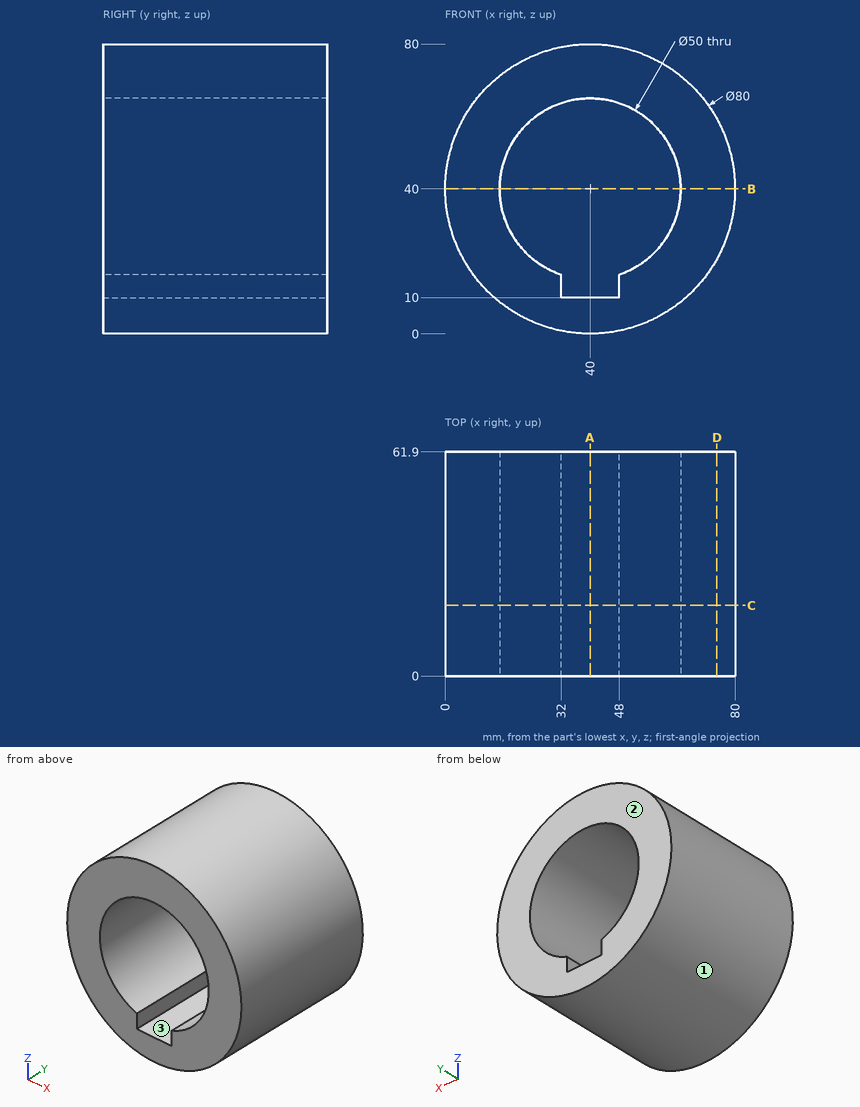
Print and shaded views of the part. All mm, measured from the part's lowest x, y and z. Coordinates: 2 decimals unless noted, no trailing zeros. Write each loop counter-clockwise with the first axis right and the second up, starting at its lowest first coordinate (ties: lowest second). Pieces come first, ordered by that corner, then holes.
(1) Cut at A-A, the plane x = 40. List the corners of the cut face in (y, z).
(2) Cut at D-D, the plane x = 75. List the corners of the cut face in (y, z).
(3) Drill centre lines: probe 1 along X at (y, z) = (45.5, 40); probe 2 along X at (y, z) = (14, 51); probe 3 along Z at (x, y) = (27.5, 32). Where is each one in solid material? Low to high.
(4) Two-plate mould, pull along Z, no slides. Class the marked faces 1, 2 and 3: +Z half, -Z half, draft (parallel to the pull), parting line (faces both ways), or undercut.
(5) Flat gauge pins, fed straight in: pin 1 (1.5 mm diameter, centred on y = 27, z = 25.5, fed in from +X); pin 2 (8 mm diameter, centred on x = 29, y = 46, fed in from -Z); pin 3 (10 mm diameter, centred on y = 39.5, z = 63, fed in from +X). Where does each tip first touch, or does it go through?
(6) Cut at C-C, the plane y = 19.5. List the corners of the cut face in (x, z), and give its area (3 significant figures).
(7) Cut at B-B, the plane z = 40. List the corners of the cut face in (x, y).
Geometry says:
1. outline: (0, 0) - (61.9, 0) - (61.9, 10) - (0, 10) - close; (0, 65) - (61.9, 65) - (61.9, 80) - (0, 80) - close
2. outline: (0, 20.64) - (61.9, 20.64) - (61.9, 59.36) - (0, 59.36) - close
3. probe 1: x = 0 to 15, 65 to 80
3. probe 2: x = 1.54 to 17.55, 62.45 to 78.46
3. probe 3: z = 2 to 18.35, 61.65 to 78
4. face 1: parting line
4. face 2: draft
4. face 3: undercut
5. pin 1: stops at x = 77.56
5. pin 2: stops at z = 0.62
5. pin 3: stops at x = 75.72
6. outline: circle Ø80 at (40, 40); hole (32, 10) - (48, 10) - (48, 16.31) arc R25 ccw (long way) to (32, 16.31) - close
6. area: 2,980 mm2
7. outline: (0, 0) - (15, 0) - (15, 61.9) - (0, 61.9) - close; (65, 0) - (80, 0) - (80, 61.9) - (65, 61.9) - close
